Input: dimensioned drawing with shaded views. Units: mm. Origin: part minimum x, y, z. Give positions to 0.01 mm unless a question says otherwise; leave off trailing zeros. Loops run counter-clockwise (first coordinate to the right, second up) from the corner with the lowest first, then second, coordinate; pieces in that order, holes last. Notation, with made-up numbers: (-12, 79.5) -> (38, 79.5) arc R18 ccw to (38, 84.5) -> close; hole circle Ø11 at (48, 44.5). An arc over 180 degrees is marked (long way). Answer in a Markdown table with one row per item. Add a question column.
1) First-contact query: P1, Ø1, axis at x = 44, z = 8, coming from the -Y side; P2, Ø1.5, axis at y = 4, z = 40, coming from the -X side; P3, Ø6, axis at x = 50.5, y = 5.5, coming from the -Z side (1 decimal); P4, Ø6, axis at y = 8.5, z = 51, coming from the -X side. Flat tips, straight axial feed; report the tip coordinate or a pass-through.
2) Section query A-A (z = 31.5). Return the cut outline in (x, y).
3) Line query: line 1 (X direction, y = 2.5, z = 31.5); line 2 (Z direction, x = 13, y = 8.75) (1 decimal); line 3 (X direction, y = 7, z = 12) (1 decimal). Output: solid intervals per line, ascending. Write a range as from..to.
4) Section query D-D (x = 16). Return the cut outline in (y, z) (1 decimal), plus the area to 3 significant figures.
5) Section query C-C (z = 43.5). Return the cut outline in (x, y) (1 decimal).
6) Section query B-B (x = 31.5). Return the cut outline in (y, z).
7) Draft query along X for the marked faces 1, 2 and 3. Return one class per face: +X half, -X half, draft (parallel to the pull), parting line (faces both ways), or undercut.
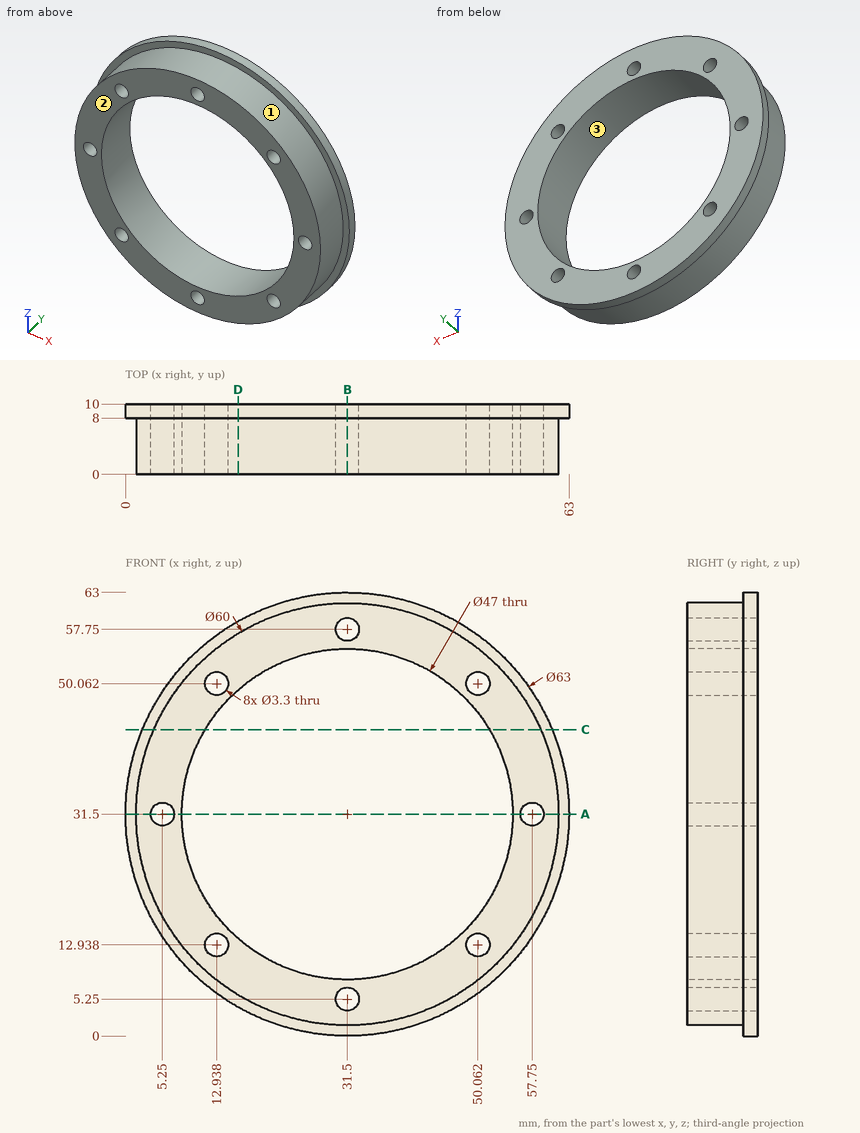
Evaluation:
| question | item | result |
|---|---|---|
| 1 | P1 | y = 0 |
| 1 | P2 | x = 2.52 |
| 1 | P3 | z = 5.2 |
| 1 | P4 | x = 4.67 |
| 2 | outline | (0, 8) -> (1.5, 8) -> (1.5, 0) -> (3.6, 0) -> (3.6, 10) -> (0, 10) -> close; (6.9, 0) -> (8, 0) -> (8, 10) -> (6.9, 10) -> close; (55, 0) -> (56.1, 0) -> (56.1, 10) -> (55, 10) -> close; (59.4, 0) -> (61.5, 0) -> (61.5, 8) -> (63, 8) -> (63, 10) -> (59.4, 10) -> close |
| 3 | line 1 | 1.5..3.6, 6.9..8, 55..56.1, 59.4..61.5 |
| 3 | line 2 | 6..11.3, 14.6..17, 46..48.4, 51.7..57 |
| 3 | line 3 | 8.7..11.6, 14.3..18.4, 44.6..48.7, 51.4..54.3 |
| 4 | outline | (0, 5.8) -> (8, 5.8) -> (8, 4.1) -> (10, 4.1) -> (10, 13.8) -> (0, 13.8) -> close; (0, 49.2) -> (10, 49.2) -> (10, 58.9) -> (8, 58.9) -> (8, 57.2) -> (0, 57.2) -> close |
| 4 | area | 167 mm² |
| 5 | outline | (2.4, 8) -> (4, 8) -> (4, 0) -> (11.3, 0) -> (11.3, 10) -> (2.4, 10) -> close; (51.7, 0) -> (59, 0) -> (59, 8) -> (60.6, 8) -> (60.6, 10) -> (51.7, 10) -> close |
| 6 | outline | (0, 1.5) -> (8, 1.5) -> (8, 0) -> (10, 0) -> (10, 3.6) -> (0, 3.6) -> close; (0, 6.9) -> (10, 6.9) -> (10, 8) -> (0, 8) -> close; (0, 55) -> (10, 55) -> (10, 56.1) -> (0, 56.1) -> close; (0, 59.4) -> (10, 59.4) -> (10, 63) -> (8, 63) -> (8, 61.5) -> (0, 61.5) -> close |
| 7 | face 1 | parting line |
| 7 | face 2 | draft |
| 7 | face 3 | undercut |
